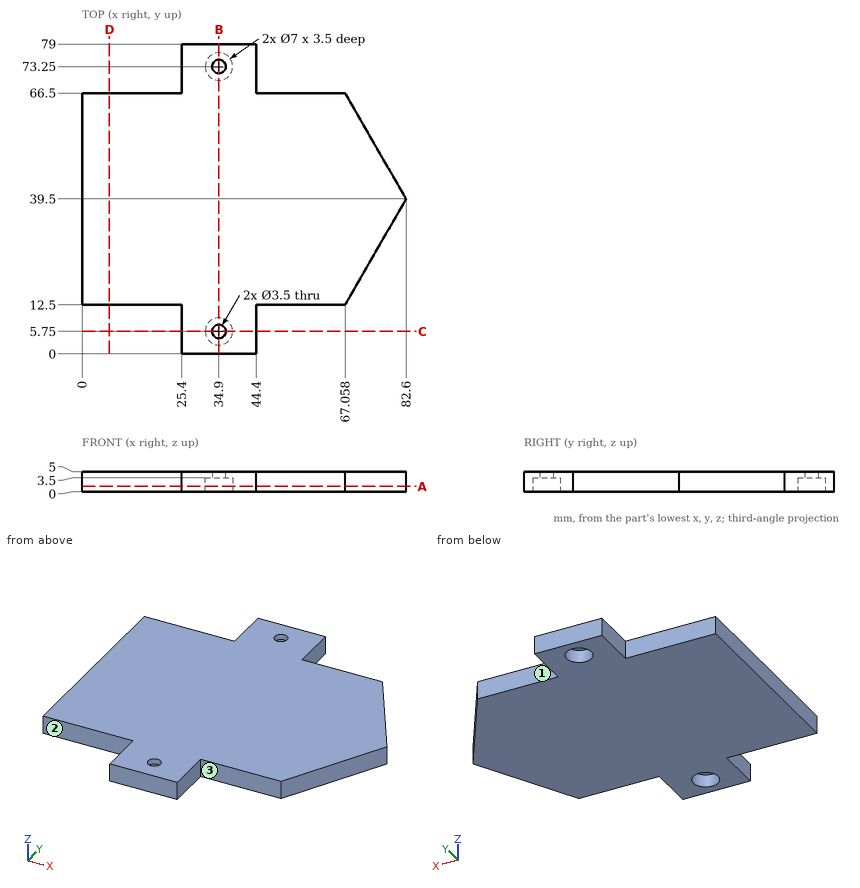
The drawing under review shows one solid part. Ordinate dimensions are in mm from its lowest x, y, z. A direction names the side the tool comes from. Give positions to 0.01 mm unless a question says otherwise; leave off trailing zeros. Write each loop counter-clockwise with the first axis right and the second up, starting at its lowest first coordinate (ties: lowest second). Pieces come first, ordered by that corner, then holes. Notation, with made-up numbers: (32.25, 57.5) -> (66.25, 57.5) arc R35 cw to (66.25, 94.5) -> close; hole circle Ø2 at (19.25, 12.5). An arc over 180 degrees is marked (long way). Put each result on its own line as item: value.
(1) To check wall thickness, follow probe 1 along Y at (x, z) = (34.9, 1.25); probe 2 along X at (y, z) = (5.75, 1.1); probe 3 along X at (y, z) = (73.25, 4). State the ranges of each line that lie inside material, in increasing order. Write a range as from..to.
Results are:
probe 1: 0..2.25, 9.25..69.75, 76.75..79
probe 2: 25.4..31.4, 38.4..44.4
probe 3: 25.4..33.15, 36.65..44.4
(2) We need section B-B, the plane x = 34.9. Give the boundary of the cut face in (y, z).
Results are:
outline: (0, 0) -> (2.25, 0) -> (2.25, 3.5) -> (4, 3.5) -> (4, 5) -> (0, 5) -> close; (7.5, 3.5) -> (9.25, 3.5) -> (9.25, 0) -> (69.75, 0) -> (69.75, 3.5) -> (71.5, 3.5) -> (71.5, 5) -> (7.5, 5) -> close; (75, 3.5) -> (76.75, 3.5) -> (76.75, 0) -> (79, 0) -> (79, 5) -> (75, 5) -> close
(3) We need section C-C, the plane y = 5.75. Give the boundary of the cut face in (x, z).
Results are:
outline: (25.4, 0) -> (31.4, 0) -> (31.4, 3.5) -> (33.15, 3.5) -> (33.15, 5) -> (25.4, 5) -> close; (36.65, 3.5) -> (38.4, 3.5) -> (38.4, 0) -> (44.4, 0) -> (44.4, 5) -> (36.65, 5) -> close
(4) Tool access review of the marked faces 1, 2 and 3: name each direction out of +Z, -Z, +X, -X, +Y, -Y from which nothing blocks a thin tool from reaching the whole face with its end or side.
Results are:
face 1: +Z, -Z, +X, +Y
face 2: +Z, -Z, -X, -Y
face 3: +Z, -Z, +X, -Y
(5) For pin 1 Ø6.5 at (x, y) = (34.9, 5.75) entering from +Z; pin 2 Ø4.5 at (x, y) = (34.9, 73.25) entering from -Z; pin 3 Ø1.5 at (x, z) = (53.5, 4.5) entering from -Y; pin 4 Ø3 at (x, z) = (69, 3) entering from -Y (1 decimal), all flat-tipped, find the tip position at first contact; note any pin that passes through.
Results are:
pin 1: z = 5
pin 2: z = 3.5
pin 3: y = 12.5
pin 4: y = 13.3
(6) We need section A-A, the plane z = 1.3. Give the boundary of the cut face in (x, y), and give its area (3 significant figures).
Results are:
outline: (0, 12.5) -> (25.4, 12.5) -> (25.4, 0) -> (44.4, 0) -> (44.4, 12.5) -> (67.06, 12.5) -> (82.6, 39.5) -> (67.06, 66.5) -> (44.4, 66.5) -> (44.4, 79) -> (25.4, 79) -> (25.4, 66.5) -> (0, 66.5) -> close; hole circle Ø7 at (34.9, 5.75); hole circle Ø7 at (34.9, 73.25)
area: 4,440 mm²
(7) We need section D-D, the plane x = 7. Give the boundary of the cut face in (y, z).
Results are:
outline: (12.5, 0) -> (66.5, 0) -> (66.5, 5) -> (12.5, 5) -> close
